```python
from build123d import *

# Parameters (mm, degrees)
SKETCH013_W     = 166
SKETCH013_H     = 266
PAD010_DEPTH    = 4
SKETCH017_W     = 26
SKETCH017_H     = 40
POCKET002_DEPTH = 631.146916
SKETCH018_W     = 40
SKETCH018_H     = 30
POCKET003_DEPTH = 4.001
POCKET012_DEPTH = 4.001


with BuildPart() as part:
    # Sketch013 (on DatumPlane) → Pad010 (new body)
    with BuildSketch(Plane(origin=(-31.154728, 0, 47), x_dir=(0, -1, 0), z_dir=(0, 0, -1))):
        with Locations((0, -31.154728)):
            Rectangle(SKETCH013_W, SKETCH013_H)
    extrude(amount=PAD010_DEPTH)

    # Sketch017 (on Face5 of Pad010) → Pocket002 (cut, through all)
    with BuildSketch(Plane(origin=(-31.154728, 0, 47), x_dir=(0, -1, 0), z_dir=(0, 0, 1))):
        with Locations((-92, 111.154728)):
            Rectangle(SKETCH017_W, SKETCH017_H)
        with Locations((-92, 31.154728)):
            Rectangle(SKETCH017_W, SKETCH017_H)
        with Locations((-92, -48.845272)):
            Rectangle(SKETCH017_W, SKETCH017_H)
    pocket002 = extrude(amount=-POCKET002_DEPTH, mode=Mode.SUBTRACT)

    # Mirrored004: Pocket002 across Sketch017 V_Axis
    add(pocket002.mirror(Plane(origin=(-31.154728, 0, 47), x_dir=(0, 0, 1), z_dir=(0, -1, 0))), mode=Mode.SUBTRACT)

    # Sketch018 (on Face4 of Mirrored004) → Pocket003 (cut, through all)
    with BuildSketch(Plane(origin=(-31.154728, 0, 47), x_dir=(0, -1, 0), z_dir=(0, 0, 1))):
        with Locations((-40, -112.845272)):
            Rectangle(SKETCH018_W, SKETCH018_H)
        with Locations((40, -112.845272)):
            Rectangle(SKETCH018_W, SKETCH018_H)
    extrude(amount=-POCKET003_DEPTH, mode=Mode.SUBTRACT)

    # Sketch029 (on Face2 of Pocket003) → Pocket012 (cut, through all)
    with BuildSketch(Plane(origin=(-31.154728, 0, 47), x_dir=(0, -1, 0), z_dir=(0, 0, 1))):
        with BuildLine():
            Line((-63, 154.154728), (63, 154.154728))
            ThreePointArc((73, 144.154728), (70.071068, 151.225796), (63, 154.154728))
            Line((73, 144.154728), (73, -81.845272))
            ThreePointArc((63, -91.845272), (70.071068, -88.91634), (73, -81.845272))
            Line((63, -91.845272), (-51, -91.845272))
            ThreePointArc((-61, -81.845272), (-58.071068, -88.91634), (-51, -91.845272))
            Line((-61, -81.845272), (-61, -31.845272))
            ThreePointArc((-61, -31.845272), (-62.6334, -26.368047), (-67, -22.680121))
            ThreePointArc((-73, -13.514969), (-71.3666, -18.992195), (-67, -22.680121))
            Line((-73, -13.514969), (-73, 144.154728))
            ThreePointArc((-63, 154.154728), (-70.071068, 151.225796), (-73, 144.154728))
        make_face()
    extrude(amount=-POCKET012_DEPTH, mode=Mode.SUBTRACT)


solid = part.part
```
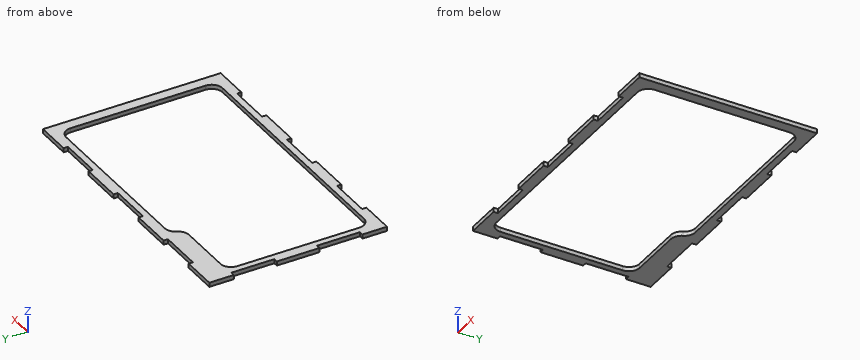
Geometry: final body of the model. Coordinates: model frame, mm. Coordinates: 2 decimals unless noted, no trailing zeros. Write each loop counter-clockwise with the first axis right and the second up, starting at its lowest first coordinate (ties: lowest second). Pieces come first, ordered by that corner, then holes. Notation, with made-up numbers: M -24,-36 L 21,-36 A13 ccw 21,-30 Z; hole C 32.25,-13 d3. An arc over 180 degrees is marked long. Answer as CSV lines item,"result". Start each with the question number.
Q1. Line query: line 1 (Y direction, x = -112.5, z = 45.9); line 2 (Y direction, x = -62.5, z = 44.15); line 3 (X direction, y = -46.5, z = 45.1). Output: solid intervals per line, ascending. Write a range as from..to.
Q2. Cut plane A-A on y = -52. Return the cut outline in (x, z).
Q3. Cut plane B-B on x = 56.5. Return the cut outline in (y, z), then the cut area to 3 significant figures.
Q4. Pin query (flat end, axial travel): P1, Ø2, axis at x = 2.5, z = 45, coming from the -Y side; P2, Ø1.5, axis at x = -71.5, z = 45.5, coming from the +Y side. Return the tip coordinate at first contact, or that it passes through.
Findings below:
1,line 1,"y = -83..-73, 61..83"
1,line 2,"y = -79..-73, 61.01..79"
1,line 3,"x = -129..-123, 123..133"
2,outline,"M -129,43 L -123,43 L -123,47 L -129,47 Z; M 123,43 L 133,43 L 133,47 L 123,47 Z"
3,outline,"M -83,43 L -73,43 L -73,47 L -83,47 Z; M 73,43 L 83,43 L 83,47 L 73,47 Z"
3,area,"80.0 mm2"
4,P1,"stops at y = -79"
4,P2,"stops at y = 79"
